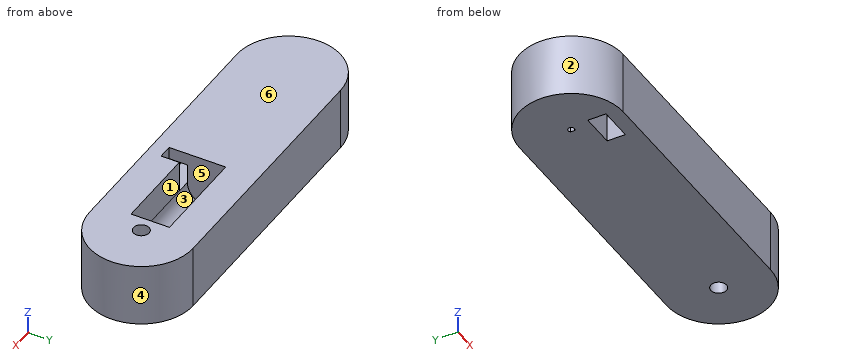
```python
from build123d import *

# Parameters (mm, degrees)
CROQUIS1_R              = 5
SALIENTE_EXTRUIR1_DEPTH = 40
CORTAR_EXTRUIR2_DEPTH   = 10
CORTAR_EXTRUIR4_DEPTH   = 20
CROQUIS6_R              = 12.2
CORTAR_EXTRUIR6_DEPTH   = 63
CROQUIS7_W              = 24.4
CROQUIS7_H              = 24.4
CORTAR_EXTRUIR9_DEPTH   = 30
CROQUIS8_W              = 12.2
CROQUIS8_H              = 11.6
CORTAR_EXTRUIR10_DEPTH  = 85
CORTAR_EXTRUIR11_REACH  = 165.418
CROQUIS9_W              = 11.6
CROQUIS9_H              = 11.6
CHAFL_N1_SIZE           = 10


with BuildPart() as part:
    # Croquis1 → Saliente-Extruir1 (new body)
    with BuildSketch(Plane.XY):
        with BuildLine():
            Line((121.972889038, 33), (-43.027110962, 33))
            ThreePointArc((-43.027110962, 33), (-76.027110962, 0), (-43.027110962, -33))
            Line((-43.027110962, -33), (121.972889038, -33))
            ThreePointArc((121.972889038, -33), (154.972889038, 0), (121.972889038, 33))
        make_face()
        with Locations((121.972889038, 0)):
            Circle(CROQUIS1_R, mode=Mode.SUBTRACT)
    extrude(amount=SALIENTE_EXTRUIR1_DEPTH)

    # Croquis1<4> → Cortar-Extruir2 (cut)
    with BuildSketch(Plane.XY):
        with BuildLine():
            Line((-41.509889959, -1.303088803), (-41.509889959, 1.303088803))
            ThreePointArc((-41.509889959, 1.303088803), (-45.027110962, 0), (-41.509889959, -1.303088803))
        make_face()
    extrude(amount=CORTAR_EXTRUIR2_DEPTH, mode=Mode.SUBTRACT)

    # Croquis5 → Cortar-Extruir4 (cut)
    with BuildSketch(Plane.XY.offset(40)):
        Polygon((111.972889038, -12.2), (111.972889038, 12.2), (48.972889038, 12.2), (48.972889038, -23.8), (57.948493167, -23.8), (57.948493167, -12.2), align=None)
    extrude(amount=-CORTAR_EXTRUIR4_DEPTH, mode=Mode.SUBTRACT)

    # Croquis6 → Cortar-Extruir6 (cut)
    with BuildSketch(Plane(origin=(48.972889038, 0, 0), x_dir=(0, 0, -1), z_dir=(1, 0, 0))):
        with Locations((-20, 0)):
            Circle(CROQUIS6_R)
        with BuildLine():
            ThreePointArc((-20, -12.2), (-32.2, 0), (-20, 12.2))
            Line((-20, 12.2), (-40, 12.2))
            Line((-40, 12.2), (-40, -12.2))
            Line((-40, -12.2), (-20, -12.2))
        make_face()
    extrude(amount=CORTAR_EXTRUIR6_DEPTH, mode=Mode.SUBTRACT)

    # Croquis7 → Cortar-Extruir9 (cut)
    with BuildSketch(Plane.ZY.offset(-111.972889038)):
        with Locations((20, 0)):
            Rectangle(CROQUIS7_W, CROQUIS7_H)
    extrude(amount=-CORTAR_EXTRUIR9_DEPTH, mode=Mode.SUBTRACT)

    # Croquis8 → Cortar-Extruir10 (cut)
    with BuildSketch(Plane(origin=(48.972889038, 0, 0), x_dir=(0, 0, -1), z_dir=(1, 0, 0))):
        with Locations((-26.1, -18)):
            Rectangle(CROQUIS8_W, CROQUIS8_H)
    extrude(amount=-CORTAR_EXTRUIR10_DEPTH, mode=Mode.SUBTRACT)

    # Croquis9 → Cortar-Extruir11 (cut, up to next)
    with BuildSketch(Plane(origin=(0, 0, 0), x_dir=(-1, 0, 0), z_dir=(0, 0, -1)), mode=Mode.PRIVATE) as cortar_extruir11_sk1:
        with Locations((30.227110962, -18)):
            Rectangle(CROQUIS9_W, CROQUIS9_H)
    cortar_extruir11_tool1 = extrude(cortar_extruir11_sk1.sketch, amount=-CORTAR_EXTRUIR11_REACH, mode=Mode.PRIVATE) & part.part
    add(cortar_extruir11_tool1.solids().sort_by_distance((-30.227111, -18, 0))[0], mode=Mode.SUBTRACT)

    # Chaflán1
    chafl_n1_edges = [part.edges().sort_by_distance(p)[0] for p in [
        (-36.027110962, -18, 0),
    ]]
    chamfer(chafl_n1_edges, length=CHAFL_N1_SIZE)


solid = part.part
```
Part model, mm, in its own coordinate system. Face numbers are marked on the shaded views. A direction names the side the tool comes from. Round coordinates to 2 decimals unless told otherwise and drop trailing zeros. Loops run counter-clockwise (first coordinate to the right, second up) from the corner with the lowest first, then second, coordinate; pieces in that order, holes last. Notation, with made-up numbers: (37.25, 4) -> (65.25, 4) arc R7 ccw to (65.25, 17) -> close; hole circle Ø8 at (81.25, 35.5). An arc over 180 degrees is marked (long way). Use one line per item in the form item = value. Start each with the question number.
Item 1: Band-saw the part on C-C (z = 17). List the corners of the cut face in (x, y).
Item 2: Two-plate mould, pull along X, no slides. Class the marked faces 4, 5 and 6: released by +X, released by -X, zero draft, split by the parting line, or undercut.
Item 3: Drill centre lines: line 1 along X through (y, z) = (0, 35.25); line 2 along X through (y, z) = (0, 3.75); line 3 along Y through (x, z) = (87.5, 36). Where is each one in solid material? Low to high.
Item 4: Drop flat-ended pins along their axis: pin 1 Ø19.5 at (y, z) = (0.5, 15.5) entering from -X; pin 2 Ø5 at (y, z) = (3, 29) entering from +X; pin 3 Ø3 at (y, z) = (23.5, 25.5) entering from +X. Give the stop position or say it passes through.
Item 5: Band-saw the part on B-B (y = -15.5). List the corners of the cut face in (x, z), plus the area to 3 significant figures.
Item 6: Band-saw the part on A-A (x = -1). List the corners of the cut face in (y, z).
Item 7: Band-saw the part on D-D (x = -28). List the corners of the cut face in (y, z), plus the area to 3 significant figures.
Item 8: Tool access for the marked faces 1, 2 and 3: list every direction of +Z, -Z, +X, -X, +Y, -Y with a clear straight run to the whole face (end or side of a thin tool).
Data:
q1.outline = (-43.03, -33) -> (121.97, -33) arc R33 ccw to (121.97, 33) -> (-43.03, 33) arc R33 ccw to start; hole (-36.03, -23.8) -> (-24.43, -23.8) -> (-24.43, -12.2) -> (-36.03, -12.2) -> close; hole (48.97, -11.83) -> (111.97, -11.83) -> (111.97, -12.2) -> (141.97, -12.2) -> (141.97, 12.2) -> (111.97, 12.2) -> (111.97, 11.83) -> (48.97, 11.83) -> close
q2.face_4 = released by +X
q2.face_5 = undercut
q2.face_6 = zero draft
q3.line_1 = -76.03 to 48.97, 111.97 to 116.97, 126.97 to 154.97
q3.line_2 = -76.03 to -45.03, -41.51 to 116.97, 126.97 to 154.97
q3.line_3 = -33 to -12.2, 12.2 to 33
q4.pin_1 = -76.03
q4.pin_2 = 154.97
q4.pin_3 = 146.57
q5.outline = (-72.16, 0) -> (-46.03, 0) -> (-36.03, 10) -> (-36.03, 32.2) -> (48.97, 32.2) -> (48.97, 40) -> (-72.16, 40) -> close; (-24.43, 0) -> (151.11, 0) -> (151.11, 40) -> (57.95, 40) -> (57.95, 20) -> (-24.43, 20) -> close
q5.area = 7,430 mm^2
q6.outline = (-33, 0) -> (33, 0) -> (33, 40) -> (-33, 40) -> close; hole (-23.8, 20) -> (-12.2, 20) -> (-12.2, 32.2) -> (-23.8, 32.2) -> close
q7.outline = (-33, 0) -> (-23.8, 0) -> (-23.8, 32.2) -> (-12.2, 32.2) -> (-12.2, 0) -> (33, 0) -> (33, 40) -> (-33, 40) -> close
q7.area = 2,270 mm^2
q8.face_1 = none
q8.face_2 = +Z, -Z, -X
q8.face_3 = +Z
